Check sheet for the modelled part. Datum: model origin and axes. Units: mm. A direction names the side the tool comes from. Give positions to 0.01 mm unless a question says otherwise; leave off trailing zeros. Loops run counter-clockwise (first coordinate to the right, second up) from the corner with the lowest first, then second, coordinate; pieces in that order, holes last.
```python
from build123d import *

# Parameters (mm, degrees)
SKETCH1_R           = 2.5
BOSS_EXTRUDE1_DEPTH = 6.5
SKETCH1_3_R         = 2
BOSS_EXTRUDE2_DEPTH = 1
SKETCH5_R           = 1
BOSS_EXTRUDE3_DEPTH = 1
SKETCH6_R           = 2
BOSS_EXTRUDE4_DEPTH = 1
SKETCH12_R          = 1.65
CUT_EXTRUDE1_DEPTH  = 5


with BuildPart() as part:
    # Sketch1 → Boss-Extrude1 (new body)
    with BuildSketch(Plane(origin=(0, 0, 0), x_dir=(1, 0, 0), z_dir=(0, 1, 0))):
        with Locations((-0.522013312, 0.511138034)):
            Circle(SKETCH1_R)
    extrude(amount=BOSS_EXTRUDE1_DEPTH)

    # Sketch1<3> → Boss-Extrude2 (add)
    with BuildSketch(Plane(origin=(0, 0, 0), x_dir=(1, 0, 0), z_dir=(0, 1, 0))):
        with Locations((-0.522013312, 0.511138034)):
            Circle(SKETCH1_3_R)
    extrude(amount=BOSS_EXTRUDE2_DEPTH)

    # Sketch5 → Boss-Extrude3 (add)
    with BuildSketch(Plane.XZ):
        with Locations((-0.522013312, -0.511138034)):
            Circle(SKETCH5_R)
    extrude(amount=BOSS_EXTRUDE3_DEPTH)

    # Sketch6 → Boss-Extrude4 (add)
    with BuildSketch(Plane.XZ.offset(1)):
        with Locations((-0.522013312, -0.511138034)):
            Circle(SKETCH6_R)
    extrude(amount=BOSS_EXTRUDE4_DEPTH)

    # Sketch12 → Cut-Extrude1 (cut)
    with BuildSketch(Plane(origin=(0, 6.5, 0), x_dir=(1, 0, 0), z_dir=(0, 1, 0))):
        with Locations((-0.522013312, 0.511138034)):
            Circle(SKETCH12_R)
    extrude(amount=-CUT_EXTRUDE1_DEPTH, mode=Mode.SUBTRACT)


solid = part.part
```
(1) Section check A-A on z = -2.35. Record the boundary of the cut face in (x, y).
(2) Section check B-B on x = -1.75. Record the boundary of the cut face in (y, z), plus the area to 3 significant figures.
(3) Section check D-D on x = 0.95. Record the boundary of the cut face in (y, z).
(4) Release check for a two-part mould opening along Y. For faces 1 (the face through (1.325, -1.493, -1.277)), 2 (the face through (1, 0, -1)), 3 (the face through (-1, 1.5, -1)) record: pulls with the +Y half, pulls with the -Y half, needs draft (parallel to the pull), parting line crosses it, or undercut.
(5) Access from +Z, -Z, +X, -X, +Y, -Y to the whole of each face (thin tool, end or side, straight path). Record for faces 4 (the face through (-0.65, -0.49, 0.48)), 5 (the face through (1.002, 4.035, 0.121)), 6 (the face through (1.863, 3.204, -1.262)).
(6) Section check C-C on z = -1.05. Record the boundary of the cut face in (x, y).
(7) Material ranges on line 1 (Y direction, x = 0.3, z = -2.25); line 2 (Z direction, x = -1.6, y = 2.25); line 3 (X direction, y = 3.5, z = -0.45), recorded low to high.
(8) Gauge pin test, flat ends, axial feed: pin 1 Ø1.2 at (x, z) = (-1.5, -0.5) entering from +Y; pin 2 Ø3 at (x, y) = (-2.5, 3) entering from +Z; pin 3 Ø1.5 at (x, y) = (-2, 1) entering from -Z. Record the tip position at first contact, or that the pin passes through.
Computed values:
1. outline: (-2.22, 0) - (1.17, 0) - (1.17, 6.5) - (-2.22, 6.5) - close; (-1.31, -2) - (0.26, -2) - (0.26, -1) - (-1.31, -1) - close
2. outline: (-2, -2.09) - (-1, -2.09) - (-1, 1.07) - (-2, 1.07) - close; (0, -2.69) - (6.5, -2.69) - (6.5, -1.61) - (1.5, -1.61) - (1.5, 0.59) - (6.5, 0.59) - (6.5, 1.67) - (0, 1.67) - close
2. area: 20.4 mm2
3. outline: (-2, -1.87) - (-1, -1.87) - (-1, 0.84) - (-2, 0.84) - close; (0, -2.53) - (6.5, -2.53) - (6.5, -1.26) - (1.5, -1.26) - (1.5, 0.23) - (6.5, 0.23) - (6.5, 1.51) - (0, 1.51) - close
4. face 1: needs draft
4. face 2: undercut
4. face 3: pulls with the +Y half
5. face 4: none
5. face 5: +Y
5. face 6: +Y, -Y
6. outline: (-2.96, 0) - (-1.36, 0) - (-1.36, -1) - (-2.45, -1) - (-2.45, -2) - (1.4, -2) - (1.4, -1) - (0.32, -1) - (0.32, 0) - (1.92, 0) - (1.92, 6.5) - (1.04, 6.5) - (1.04, 1.5) - (-2.08, 1.5) - (-2.08, 6.5) - (-2.96, 6.5) - close
7. line 1: y = -2 to -1, 0 to 6.5
7. line 2: z = -2.77 to -1.76, 0.74 to 1.74
7. line 3: x = -3.02 to -2.17, 1.13 to 1.98
8. pin 1: stops at y = 1.5
8. pin 2: stops at z = 1.94
8. pin 3: stops at z = -2.9
